Autodesk Inventor part; units mm, degrees
ref_plane "YZ Plane" through (0, 0, 0) normal (1, 0, 0) x (0, 1, 0)
ref_plane "XZ Plane" through (0, 0, 0) normal (0, 1, 0) x (-1, 0, 0)
ref_plane "XY Plane" through (0, 0, 0) normal (0, 0, 1) x (1, 0, 0)
sketch "Sketch1" plane through (0, 0, 0) normal (0, 1, 0) x (-1, 0, 0)
  circle A0 centre (0, 0) radius 27.94
  dimension "d0" = 55.88
extrude "Extrusion1" add sketch "Sketch1" along normal blind 7.62
ref_plane "Work Plane5" through (0, 21.082, 0) normal (0, 1, 0) x (1, 0, 0)
sketch "Sketch5" plane through (0, 21.082, 0) normal (0, 1, 0) x (1, 0, 0)
  line L0 (0, 0) -> (0, 2.667)
  line L1 (-3.1168, 0) -> (-1.5584, 2.6992)
  line L2 (-1.5584, 2.6992) -> (1.5584, 2.6992)
  line L3 (1.5584, 2.6992) -> (3.1168, 0)
  line L4 (3.1168, 0) -> (1.5584, -2.6992)
  line L5 (1.5584, -2.6992) -> (-1.5584, -2.6992)
  line L6 (-1.5584, -2.6992) -> (-3.1168, 0)
  dimension "d10" = 2.667
extrude "Extrusion4" cut sketch "Sketch5" against normal blind 25.4
sketch "Sketch6" plane through (0, 7.62, 0) normal (0, 1, 0) x (1, 0, 0)
  circle A0 centre (0, 0) radius 27.94
  line L0 (0, -27.94) -> (0, -26.162)
  line L1 (0, -26.162) -> (0, -24.257)
  circle A1 centre (0, -24.257) radius 1.905
  dimension "d13" = 1.778
  dimension "d14" = 1.905
extrude "Extrusion5" cut sketch "Sketch6" against normal blind 25.4 contours A1
ref_plane "Work Plane6" through (0, 21.082, 0) normal (0, 1, 0) x (1, 0, 0)
pattern_circular "Circular Pattern1" count 6 over 360 about axis through (0, 21.082, 0) along (0, 1, 0) of "Extrusion5"
sketch "Sketch8" plane through (0, 0, 0) normal (0, -1, 0) x (1, 0, 0)
  line L0 (3.1168, 0) -> (1.5584, -2.6992)
  line L1 (3.1168, 0) -> (7.4348, 0)
  line L2 (7.4348, 0) -> (8.9588, 0)
  circle A0 centre (8.9588, 0) radius 1.524
  point P0 (0, 0)
  dimension "d20" = 4.318
  dimension "d21" = 1.524
extrude "Extrusion6" cut sketch "Sketch8" against normal blind 25.4
pattern_circular "Circular Pattern2" count 4 over 360 about axis through (0, 21.082, 0) along (0, 1, 0) of "Extrusion6"
properties part number "Wheel Mount"
Work out the finished part from the listing and answer in its coordinate system (mm). A direction names the side the tool comes from. Round coordinates to 2 decimals unless told otherwise and drop trailing zeros. Write each loop counter-clockwise with the first axis right and the second up, starting at its lowest first coordinate (ties: lowest second). Pieces come first, ordered by that corner, then holes. Notation, with made-up numbers: M 11.5,68.5 L 46.5,68.5 A25 ccw 46.5,99.5 Z; hole C 76.5,73.25 d10. An arc over 180 degrees is marked long. Use a Markdown table: item, result.
1) The part is cut by section B-B on y = 3. State how many separate pieces and enclosed holes the cut face has, plus the area to 3 significant figures.
Taken from the geometry:
| item | result |
|---|---|
| separate pieces | 1 |
| enclosed holes | 11 |
| area | 2,330 mm2 |
2) The part is cut by section C-C on x = -16.5. Give the vertices of the cut face in (y, z).
Taken from the geometry:
| item | result |
|---|---|
| outline | M 0,-22.55 L 7.62,-22.55 L 7.62,22.55 L 0,22.55 Z |
3) Consider line 1 (Z direction, x = 0, y = 5.5); line 2 (X direction, y = 0.5, z = -0.5); line 3 (X direction, y = 1.25, z = 11.5). Determine where each line is inside the solid, lowest interval first. Write a range as [from, to].
Taken from the geometry:
| item | result |
|---|---|
| line 1 | z = [-27.94, -26.16], [-22.35, -10.48], [-7.43, -2.7], [2.7, 7.43], [10.48, 22.35], [26.16, 27.94] |
| line 2 | x = [-27.94, -10.4], [-7.52, -2.83], [2.83, 7.52], [10.4, 27.94] |
| line 3 | x = [-25.46, -22.81], [-19.21, 19.21], [22.81, 25.46] |
4) Determine the mould class of faces 1 (the face through (-2.35, 3.86, -1.33)), 2 (the face through (-6, 7.62, 0)), 3 (the face through (3.64, 3.76, -27.7)) for opening direction Z: pulls with the +Z half, pulls with the -Z half, needs draft (parallel to the pull), parting line crosses it, or undercut.
Taken from the geometry:
| item | result |
|---|---|
| face 1 | undercut |
| face 2 | needs draft |
| face 3 | parting line crosses it |
5) Which of the six approach directions +Z, -Z, +X, -X, +Y, -Y give full straight-line access (tool end or side, diameter ignored) to faces 4 (the face through (0, 4, 2.699)), 5 (the face through (-6, 0, 0))?
Taken from the geometry:
| item | result |
|---|---|
| face 4 | +Y, -Y |
| face 5 | +Z, -Z, +X, -X, -Y |
6) The part is cut by section A-A on x = 0. Give the vertices of the cut face in (y, z), plus the area to 3 significant figures.
Taken from the geometry:
| item | result |
|---|---|
| outline | M 0,-27.94 L 7.62,-27.94 L 7.62,-26.16 L 0,-26.16 Z; M 0,-22.35 L 7.62,-22.35 L 7.62,-10.48 L 0,-10.48 Z; M 0,-7.43 L 7.62,-7.43 L 7.62,-2.7 L 0,-2.7 Z; M 0,2.7 L 7.62,2.7 L 7.62,7.43 L 0,7.43 Z; M 0,10.48 L 7.62,10.48 L 7.62,22.35 L 0,22.35 Z; M 0,26.16 L 7.62,26.16 L 7.62,27.94 L 0,27.94 Z |
| area | 280 mm2 |
7) Flat-ended cylindrical pins translate along their axes: pin 1 (1.5 mm diameter, centred on x = -16.5, y = 6.5, fed in from +Z); pin 2 (5 mm diameter, centred on x = 21.01, z = 12.13, fed in from +Y); pin 3 (2 mm diameter, centred on y = 6.5, z = -5, fed in from -X); pin 4 (0.9 mm diameter, centred on x = 0.5, y = 4, fed in from +Z). Find the tip coordinate at first contact, or state that the pin passes through.
Taken from the geometry:
| item | result |
|---|---|
| pin 1 | stops at z = 23.08 |
| pin 2 | stops at y = 7.62 |
| pin 3 | stops at x = -27.65 |
| pin 4 | stops at z = 27.94 |
8) The part is cut by section D-D on z = -20. Give the vertices of the cut face in (x, y), plus the area to 3 significant figures.
Taken from the geometry:
| item | result |
|---|---|
| outline | M -19.51,0 L 19.51,0 L 19.51,7.62 L -19.51,7.62 Z |
| area | 297 mm2 |
